Part print with two shaded views. Sizes in mm from the minimum x, y, z corner. Give positions to 0.01 mm unless a question says otherwise; leave off trailing zeros. Write each loop counter-clockwise with the first axis right and the second up, starting at its lowest first coordinate (ties: lowest second). Pieces come first, ordered by that corner, then holes.
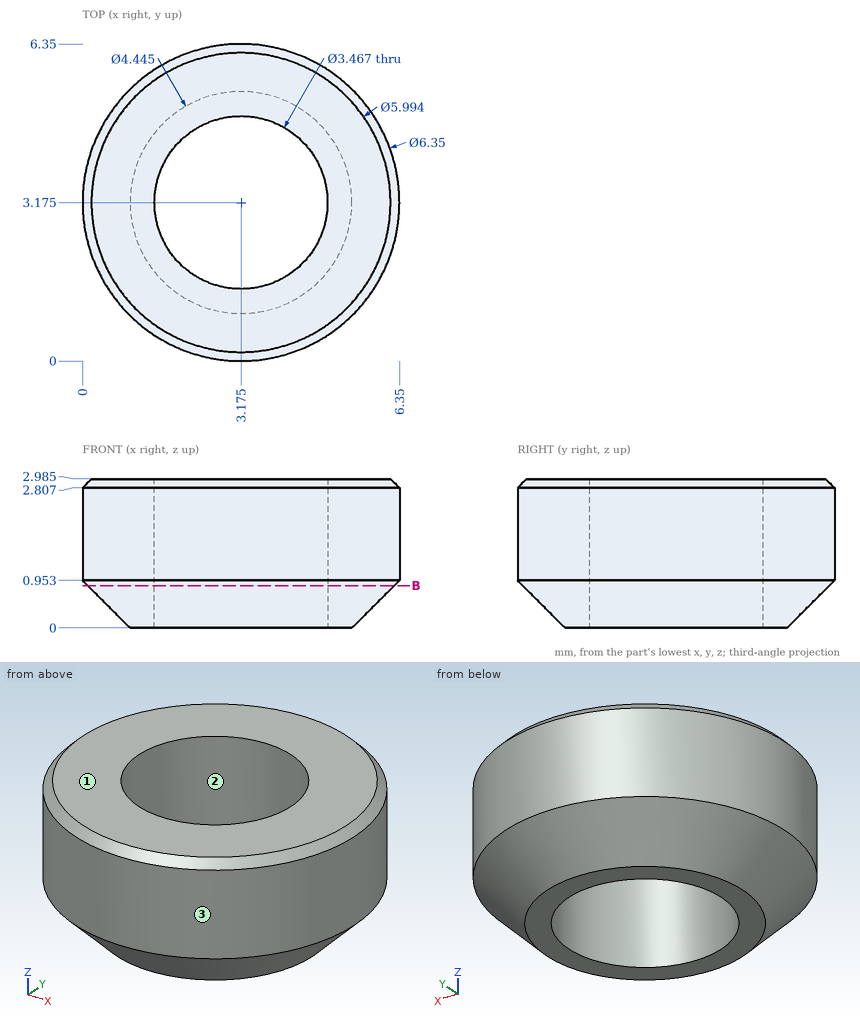
1) Pin check, flat tips, straight feed: pin 1 Ø1.5 at (x, z) = (2, 1) entering from -Y; pin 2 Ø1.5 at (y, z) = (2, 2) entering from -X; pin 3 Ø1 at (y, z) = (0.5, 0.5) entering from +X (1 decimal). Stop position of each tip, or through.
Answers follow:
pin 1: stops at y = 0.03
pin 2: stops at x = 0.03
pin 3: stops at x = 5.2
2) Saw through at B-B, the plane z = 0.85. Write the cut outline in (x, y) (1 decimal).
Answers follow:
outline: circle Ø6.1 at (3.2, 3.2); hole circle Ø3.5 at (3.2, 3.2)
3) Two-plate mould, pull along X, no slides. Class the marked faces 1, 2 and 3: +X half, -X half, draft (parallel to the pull), parting line (faces both ways), or undercut.
Answers follow:
face 1: draft
face 2: undercut
face 3: parting line
4) Wall check: L1, parallel to Y at x = 3.25, z = 2.05; L2, parallel to Y at x = 2.75, z = 1.25 (1 decimal); L3, parallel to X at y = 4.5, z = 0.3 (1 decimal). Give the ranges that are in metal, low to high.
Answers follow:
L1: y = 0 to 1.44, 4.91 to 6.35
L2: y = 0 to 1.5, 4.9 to 6.3
L3: x = 1 to 2.1, 4.3 to 5.3
